Build history of the part. All positions in model axes, mm. Face numbers are marked on the shaded views. A direction names the side the tool comes from. Give positions to 0.01 mm unless a question says otherwise; leave off trailing zeros. Order: outer loops, then holes, each group sorted by start corner. A loop starts at its lowest first (then second) coordinate and runs counter-clockwise, first axis right, second up. Notation, with made-up numbers: M 59,32 L 107,32 A26 ccw 107,54 Z; hole C -31.75,-20 d3. An arc over 180 degrees is marked long. Answer as CSV lines item,"result".
from build123d import *

# Parameters (mm, degrees)
EXTRUDE_1_DEPTH     = 16
FILLET_1_R          = 10
FILLET_2_R          = 30
EXTRUDE_2_DEPTH     = 14
SKETCH_5_R          = 9
EXTRUDE_3_DEPTH     = 9
SKETCH_7_R          = 9
CUT_EXTRUDE_2_DEPTH = 212.719153597


with BuildPart() as part:
    # Sketch 3 → Extrude 1 (new body)
    with BuildSketch(Plane(origin=(0, 0, 0), x_dir=(1, 0, 0), z_dir=(0, 1, 0))):
        with BuildLine():
            Line((0, 0), (0, 90))
            Line((0, 90), (100, 90))
            Line((100, 90), (176.45483392, 63.929741653))
            ThreePointArc((176.45483392, 63.929741653), (190, 45), (176.45483392, 26.070258347))
            Line((176.45483392, 26.070258347), (100, 0))
            Line((100, 0), (0, 0))
        make_face()
    extrude(amount=EXTRUDE_1_DEPTH)

    # Fillet 1
    fillet_1_edges = [part.edges().sort_by_distance(p)[0] for p in [
        (0, 8, 0),
        (0, 8, -90),
    ]]
    fillet(fillet_1_edges, radius=FILLET_1_R)

    # Fillet 2
    fillet_2_edges = [part.edges().sort_by_distance(p)[0] for p in [
        (100, 8, -90),
        (100, 8, 0),
    ]]
    fillet(fillet_2_edges, radius=FILLET_2_R)

    # Sketch 4 → Extrude 2 (add)
    with BuildSketch(Plane(origin=(0, 16, 0), x_dir=(1, 0, 0), z_dir=(0, 1, 0))):
        with BuildLine():
            Line((32, 75), (68, 75))
            ThreePointArc((68, 75), (76.485281374, 71.485281374), (80, 63))
            Line((80, 63), (80, 27))
            ThreePointArc((80, 27), (76.485281374, 18.514718626), (68, 15))
            Line((68, 15), (32, 15))
            ThreePointArc((32, 15), (23.514718626, 18.514718626), (20, 27))
            Line((20, 27), (20, 63))
            ThreePointArc((20, 63), (23.514718626, 71.485281374), (32, 75))
        make_face()
        with BuildLine():
            Line((28, 63), (28, 49))
            Line((28, 49), (32, 49))
            Line((32, 49), (32, 45))
            Line((32, 45), (32, 41))
            Line((32, 41), (28, 41))
            Line((28, 41), (28, 27))
            ThreePointArc((28, 27), (29.171572875, 24.171572875), (32, 23))
            Line((32, 23), (68, 23))
            ThreePointArc((68, 23), (70.828427125, 24.171572875), (72, 27))
            Line((72, 27), (72, 41))
            Line((72, 41), (68, 41))
            Line((68, 41), (68, 45))
            Line((68, 45), (68, 49))
            Line((68, 49), (72, 49))
            Line((72, 49), (72, 63))
            ThreePointArc((72, 63), (70.828427125, 65.828427125), (68, 67))
            Line((68, 67), (32, 67))
            ThreePointArc((32, 67), (29.171572875, 65.828427125), (28, 63))
        make_face(mode=Mode.SUBTRACT)
    extrude(amount=EXTRUDE_2_DEPTH)

    # Sketch 5 → Extrude 3 (add)
    with BuildSketch(Plane(origin=(0, 16, 0), x_dir=(1, 0, 0), z_dir=(0, 1, 0))):
        with BuildLine():
            ThreePointArc((113.54516608, 26.070258347), (100, 45), (113.54516608, 63.929741653))
            Line((113.54516608, 63.929741653), (176.45483392, 63.929741653))
            ThreePointArc((176.45483392, 63.929741653), (190, 45), (176.45483392, 26.070258347))
            Line((176.45483392, 26.070258347), (113.54516608, 26.070258347))
        make_face()
        with Locations(Location((120, 45, 0), (0, 0, 270))):
            Circle(SKETCH_5_R, mode=Mode.SUBTRACT)
        with Locations(Location((170, 45, 0), (0, 0, 270))):
            Circle(SKETCH_5_R, mode=Mode.SUBTRACT)
    extrude(amount=EXTRUDE_3_DEPTH)

    # Sketch 7 → Cut-Extrude 2 (cut, through all)
    with BuildSketch(Plane(origin=(0, 25, 0), x_dir=(1, 0, 0), z_dir=(0, 1, 0))):
        with Locations(Location((120, 45, 0), (0, 0, 270))):
            Circle(SKETCH_7_R)
        with Locations(Location((170, 45, 0), (0, 0, 270))):
            Circle(SKETCH_7_R)
    extrude(amount=-CUT_EXTRUDE_2_DEPTH, mode=Mode.SUBTRACT)


solid = part.part
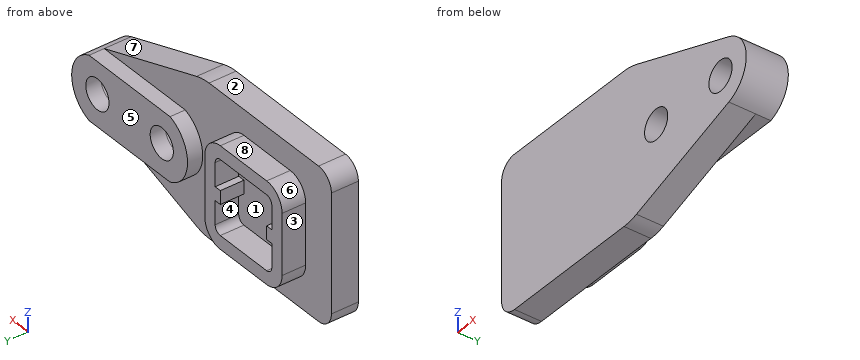
Item 1: Pull direction Z, two halves, no side cores. Call the marked faces 1, 2 and 3: released by +Z, released by -Z, zero draft, split by the parting line, or undercut.
Geometry says:
face 1,"undercut"
face 2,"released by +Z"
face 3,"zero draft"
Item 2: Band-saw the part on A-A (z = -45). Give the cut face in (x, y).
Geometry says:
outline,"M 0,0 L 111,0 L 111,25 L 100,25 L 100,16 L 80,16 L 80,30 L 68,30 L 68,16 L 32,16 L 32,30 L 20,30 L 20,16 L 0,16 Z; M 129,0 L 161,0 L 161,25 L 129,25 Z; M 179,0 L 190,0 L 190,25 L 179,25 Z"
Item 3: Band-saw the part on D-D (y = 10.75). Give the cut face in (x, z), and give its area (3 significant figures).
Geometry says:
outline,"M 0,-80 A10 ccw 10,-90 L 95.03,-90 A30 ccw 104.71,-88.39 L 176.45,-63.93 A20 ccw 176.45,-26.07 L 104.71,-1.61 A30 ccw 95.03,0 L 10,0 A10 ccw 0,-10 Z; hole C 120,-45 d18; hole C 170,-45 d18"
area,"13,700 mm2"
Item 4: Band-saw the part on C-C (x = 120). Give the cut face in (y, z), and give its area (3 significant figures).
Geometry says:
outline,"M 0,-83.18 L 16,-83.18 L 16,-63.93 L 25,-63.93 L 25,-54 L 0,-54 Z; M 0,-36 L 25,-36 L 25,-26.07 L 16,-26.07 L 16,-6.82 L 0,-6.82 Z"
area,"1,110 mm2"
Item 5: 3-axis set-ups, long thin cutter, end or side, ignore diameter. For the marked faces 4, 5, 6, 7 and 8: which of +Z, -Z, +X, -X, +Y, -Y reach the whole face in a straight line?
Geometry says:
face 4,"+Y"
face 5,"+Z, -Z, +X, +Y"
face 6,"+Z, -X, +Y"
face 7,"+Z, +X, +Y, -Y"
face 8,"+Z, +X, -X, +Y"
Item 6: Probe line 1 along X through (y, z) = (12.25, -45); line 2 along Z through (x, y) = (39.5, 26.25); line 3 along X through (y, z) = (11, -41). List the from-to ranges inside material, lowest first. Write a range as from..to.
Geometry says:
line 1,"x = 0..111, 129..161, 179..190"
line 2,"z = -75..-67, -23..-15"
line 3,"x = 0..111.94, 128.06..161.94, 178.06..189.6"
Item 7: Drop flat-ended pins along their axis: pin 1 (14.5 mm diameter, centred on x = 120, z = -45, fed in from -Y); pin 2 (11 mm diameter, centred on y = 24.5, z = -55, fed in from -X); pin 3 (7 mm diameter, centred on y = 25.5, z = -33, fed in from +X); pin 4 (15.5 mm diameter, centred on x = 54, y = 22.5, fed in from -Z). Give the stop position or say it passes through.
Geometry says:
pin 1,"passes through"
pin 2,"stops at x = 20"
pin 3,"stops at x = 188.09"
pin 4,"stops at z = -90"
Item 8: Band-saw the part on B-B (y = 28). Give the cut face in (x, z).
Geometry says:
outline,"M 20,-63 A12 ccw 32,-75 L 68,-75 A12 ccw 80,-63 L 80,-27 A12 ccw 68,-15 L 32,-15 A12 ccw 20,-27 Z; hole M 28,-63 A4 ccw 32,-67 L 68,-67 A4 ccw 72,-63 L 72,-49 L 68,-49 L 68,-41 L 72,-41 L 72,-27 A4 ccw 68,-23 L 32,-23 A4 ccw 28,-27 L 28,-41 L 32,-41 L 32,-49 L 28,-49 Z"
